Part model, mm, in its own coordinate system. A direction names the side the tool comes from. Round coordinates to 2 decimals unless told otherwise and drop trailing zeros. Write each loop counter-clockwise with the first axis right and the second up, starting at its lowest first coordinate (ties: lowest second). Pieces come first, ordered by that corner, then holes.
1) Flat gauge pins, fed straight in: pin 1 (2.5 mm diameter, centred on x = 3.5, y = 0, fed in from -Z); pin 2 (3.5 mm diameter, centred on x = -10, y = 1, fed in from +Z); pin 3 (0.9 mm diameter, centred on x = 8.5, z = -2, fed in from +Y); pin 4 (3.5 mm diameter, centred on x = 9, z = -2, fed in from -Y). Where does each tip first touch, or does it go through?
2) Drill centre lines: L1, parallel to Y at x = -8, z = -2.25; L2, parallel to X at y = -1.75, z = -2; L3, parallel to Z at x = -1.75, y = -3. Where is each one in solid material? Low to high.
3) Pull direction Y, two halves, no side cores. Call faces 4 (the flat face through (0, 0, 2.5)), 5 (the flat face through (-1.7, 0, -2)), 6 (the flat face through (0, 3.8, 1)): +Y half, -Y half, draft (parallel to the pull), parting line (faces both ways), or undercut.
4) Which spindle directions (+Z, -Z, +X, -X, +Y, -Y) get a long thin tool onto all of the face, cutting with end or side? Do faces 1 (the flat face through (11.5, 0.1, 0)), 2 (the flat face through (-8, 0, 0)), 3 (the flat face through (0, -2, -3)). Say none if no direction does.
5) Saw through at A-A on z = -1.25. Write the cut outline in (x, y), and give its area (3 significant figures).
```python
from build123d import *

# Parameters (mm, degrees)
PAD036_DEPTH    = 2.5
PAD037_DEPTH    = 3
SKETCH094_W     = 3.4
SKETCH094_H     = 2.2
POCKET015_DEPTH = 3


with BuildPart() as part:
    # Sketch066 → Pad036 (new body)
    with BuildSketch(Plane.XY):
        with BuildLine():
            ThreePointArc((-7.5, 3.8), (-11.3, 0), (-7.5, -3.8))
            Line((-7.5, -3.8), (7.5, -3.8))
            ThreePointArc((7.5, -3.8), (11.3, 0), (7.5, 3.8))
            Line((7.5, 3.8), (-7.5, 3.8))
        make_face()
    extrude(amount=PAD036_DEPTH)

    # Sketch067 → Pad037 (join)
    with BuildSketch(Plane.XY):
        with BuildLine():
            Line((-11.75, 3.75), (11.75, 3.75))
            ThreePointArc((12.75, 2.75), (12.457107, 3.457107), (11.75, 3.75))
            Line((12.75, 2.75), (12.75, -2.75))
            ThreePointArc((11.75, -3.75), (12.457107, -3.457107), (12.75, -2.75))
            Line((11.75, -3.75), (-11.75, -3.75))
            ThreePointArc((-12.75, -2.75), (-12.457107, -3.457107), (-11.75, -3.75))
            Line((-12.75, 2.75), (-12.75, -2.75))
            ThreePointArc((-11.75, 3.75), (-12.457107, 3.457107), (-12.75, 2.75))
        make_face()
    extrude(amount=-PAD037_DEPTH)

    # Sketch094 (on Face16 of Pad037) → Pocket015 (cut)
    with BuildSketch(Plane(origin=(0, 0, -3), x_dir=(1, 0, 0), z_dir=(0, 0, -1))):
        with Locations((-8.4, 0)):
            Rectangle(SKETCH094_W, SKETCH094_H)
        with Locations((8.4, 0)):
            Rectangle(SKETCH094_W, SKETCH094_H)
        Rectangle(SKETCH094_W, SKETCH094_H)
        with BuildLine():
            ThreePointArc((-2.7, 1.5), (-4.2, 3), (-5.7, 1.5))
            Line((-5.7, 1.5), (-5.7, -1.5))
            ThreePointArc((-5.7, -1.5), (-4.2, -3), (-2.7, -1.5))
            Line((-2.7, -1.5), (-2.7, 1.5))
        make_face()
        with BuildLine():
            ThreePointArc((5.7, 1.5), (4.2, 3), (2.7, 1.5))
            Line((2.7, -1.5), (2.7, 1.5))
            ThreePointArc((2.7, -1.5), (4.2, -3), (5.7, -1.5))
            Line((5.7, 1.5), (5.7, -1.5))
        make_face()
    extrude(amount=-POCKET015_DEPTH, mode=Mode.SUBTRACT)


with BuildPart() as part_1:
    # Body050 placement: moved
    add(part.part.moved(Location((0, 0, 12.5))))


with BuildPart() as part_2:
    # Clone017 placement: moved
    add(part_1.part.moved(Location((0, 0, -12.5))))

    # Sketch095 → Revolution003 (revolve)
    with BuildSketch(Plane(origin=(7.5, 0, 2.5), x_dir=(1, 0, 0), z_dir=(0, -1, 0))):
        with BuildLine():
            Line((0, 2.5), (0, 0))
            Line((0, 0), (3.8, 0))
            ThreePointArc((3.8, 0), (2.274313, 1.818956), (0, 2.5))
        make_face()
    revolution003 = revolve(axis=Axis((7.5, 0, 2.5), (0, 0, 1)))

    # Mirrored014: Revolution003 across YZ
    add(revolution003.mirror(Plane.YZ))


solid = part_2.part
```
Completed:
1. pin 1: stops at z = -3
1. pin 2: stops at z = 4.89
1. pin 3: stops at y = 3.75
1. pin 4: stops at y = -3.75
2. L1: y = -3.75 to -1.1, 1.1 to 3.75
2. L2: x = -12.75 to -5.68, -2.72 to 2.72, 5.68 to 12.75
2. L3: z = -3 to 2.5
3. face 4: draft
3. face 5: undercut
3. face 6: +Y half
4. face 1: +Z, +X
4. face 2: -Z
4. face 3: -Z, +X, -X, +Y, -Y
5. outline: (-12.75, -2.75) arc R1 ccw to (-11.75, -3.75) - (11.75, -3.75) arc R1 ccw to (12.75, -2.75) - (12.75, 2.75) arc R1 ccw to (11.75, 3.75) - (-11.75, 3.75) arc R1 ccw to (-12.75, 2.75) - close; hole (-10.1, -1.1) - (-6.7, -1.1) - (-6.7, 1.1) - (-10.1, 1.1) - close; hole (-5.7, -1.5) arc R1.5 ccw to (-2.7, -1.5) - (-2.7, 1.5) arc R1.5 ccw to (-5.7, 1.5) - close; hole (-1.7, -1.1) - (1.7, -1.1) - (1.7, 1.1) - (-1.7, 1.1) - close; hole (2.7, -1.5) arc R1.5 ccw to (5.7, -1.5) - (5.7, 1.5) arc R1.5 ccw to (2.7, 1.5) - close; hole (6.7, -1.1) - (10.1, -1.1) - (10.1, 1.1) - (6.7, 1.1) - close
5. area: 136 mm2
